Geometry: final body of the model. Coordinates: model frame, mm. Face numbers are marked on the shaded views. A direction names the side the tool comes from. Give positions to 0.01 mm unless a question says otherwise; leave off trailing zeros. Write each loop counter-clockwise with the first axis right and the second up, starting at its lowest first coordinate (ties: lowest second). Pieces come first, ordered by that corner, then holes.
Q1. Section C-C (y = 1.5). Return the cut outline in (x, z).
Q2. Mould query, pull axis X, two halves, no side actions, for the marked faces 6, 7, 8 and 9. Classes: +X half, -X half, draft (parallel to the pull), parting line (faces both ways), or undercut.
Q3. Section B-B (x = 3.5). Return the cut outline in (y, z), plus the area to 3 significant figures.
Q4. Section D-D (x = 18.5). Return the cut outline in (y, z), plus the area to 3 significant figures.
Q5. Line query: line 1 (Y direction, x = -9, z = 5.5); line 2 (X direction, y = -7, z = 0.25); line 3 (X direction, y = -10, z = 3.25). Output: solid intervals per line, ascending.
Q6. Pin query (flat end, axial travel): pin 1 Ø1 at (x, z) = (25.5, 3.5) entering from +Y; pin 2 Ø2 at (y, z) = (-25.5, -0.5) entering from -X; pin 3 Ø10 at (x, z) = (-21.5, 5) entering from -Y. Return the tip coordinate at first contact, or that it passes through.
Q7. Section A-A (z = 3.5). Return the cut outline in (x, y), plus the area to 3 significant figures.
Q8. Reachability of the marked faces 1, 2, 3, 4 and 5 from +Z, -Z, +X, -X, +Y, -Y: full face, straight path, thin tool, end or side. Return the list, or none.
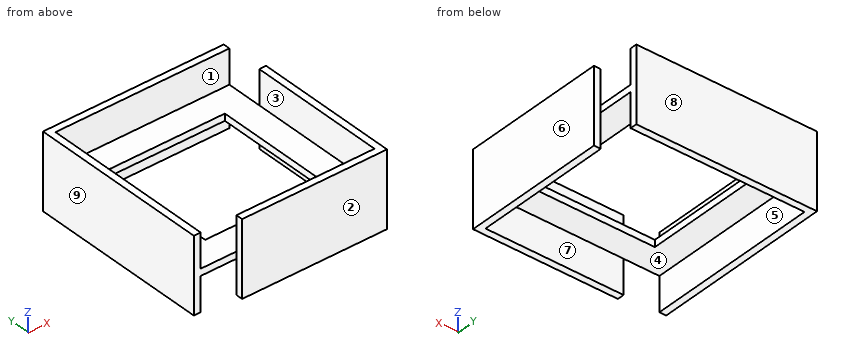
from build123d import *

# Parameters (mm, degrees)
F1_DEPTH = 12
F0_W     = 35
F0_H     = 35
F2_DEPTH = 2
F0_R     = 5
F3_DEPTH = 10


with BuildPart() as f1:
    # F0 (on Top) → F1 (new body)
    with BuildSketch(Plane.XY):
        Polygon((24.28125, 28.71875), (-28.71875, 28.71875), (-28.71875, -24.28125), (-26.71875, -24.28125), (-26.71875, 26.71875), (24.28125, 26.71875), align=None)
    extrude(amount=F1_DEPTH)



with BuildPart() as f1b:
    # F0 (on Top) → F1, piece 2 (new body)
    with BuildSketch(Plane.XY):
        Polygon((26.28125, -26.28125), (26.28125, 16.21875), (24.28125, 16.21875), (24.28125, -24.28125), (-16.21875, -24.28125), (-16.21875, -26.28125), align=None)
    extrude(amount=F1_DEPTH)


with BuildPart() as f1_1:
    add(f1.part)

    add(f1b.part)  # F2 merges F1b
    # F0 (on Top) → F2 (join)
    with BuildSketch(Plane.XY):
        Polygon((24.28125, 18.71875), (24.28125, 26.71875), (-26.71875, 26.71875), (-26.71875, -24.28125), (-18.71875, -24.28125), (-16.21875, -24.28125), (24.28125, -24.28125), (24.28125, 16.21875), align=None)
        with Locations((-1.21875, 1.21875)):
            Rectangle(F0_W, F0_H, mode=Mode.SUBTRACT)
    extrude(amount=F2_DEPTH)

    # F0 (on Top) → F3 (join)
    with BuildSketch(Plane.XY):
        Polygon((24.28125, 28.71875), (-28.71875, 28.71875), (-28.71875, -24.28125), (-26.71875, -24.28125), (-26.71875, 26.71875), (24.28125, 26.71875), align=None)
        Polygon((26.28125, -26.28125), (26.28125, 16.21875), (24.28125, 16.21875), (24.28125, -24.28125), (-16.21875, -24.28125), (-16.21875, -26.28125), align=None)
    extrude(amount=-F3_DEPTH)


with BuildPart() as f2:
    # F0 (on Top) → F2, piece 2 (new body)
    with BuildSketch(Plane.XY):
        with Locations((-1.21875, 1.21875)):
            Circle(F0_R)
    extrude(amount=F2_DEPTH)


solid = f1_1.part
Computed:
1. outline: (-28.72, -10) - (-26.72, -10) - (-26.72, 0) - (-18.72, 0) - (-18.72, 2) - (-26.72, 2) - (-26.72, 12) - (-28.72, 12) - close; (16.28, 0) - (24.28, 0) - (24.28, -10) - (26.28, -10) - (26.28, 12) - (24.28, 12) - (24.28, 2) - (16.28, 2) - close
2. face 6: +X half
2. face 7: undercut
2. face 8: draft
2. face 9: -X half
3. outline: (-26.28, -10) - (-24.28, -10) - (-24.28, 0) - (-16.28, 0) - (-16.28, 2) - (-24.28, 2) - (-24.28, 12) - (-26.28, 12) - close; (18.72, 0) - (26.72, 0) - (26.72, -10) - (28.72, -10) - (28.72, 12) - (26.72, 12) - (26.72, 2) - (18.72, 2) - close
3. area: 120 mm2
4. outline: (-26.28, -10) - (-24.28, -10) - (-24.28, 0) - (26.72, 0) - (26.72, -10) - (28.72, -10) - (28.72, 12) - (26.72, 12) - (26.72, 2) - (-24.28, 2) - (-24.28, 12) - (-26.28, 12) - close
4. area: 190 mm2
5. line 1: y = -26.28 to -24.28, 26.72 to 28.72
5. line 2: x = -28.72 to -18.72, 16.28 to 26.28
5. line 3: x = -28.72 to -26.72, 24.28 to 26.28
6. pin 1: stops at y = 16.22
6. pin 2: stops at x = -16.22
6. pin 3: stops at y = -24.28
7. outline: (-28.72, -24.28) - (-26.72, -24.28) - (-26.72, 26.72) - (24.28, 26.72) - (24.28, 28.72) - (-28.72, 28.72) - close; (-16.22, -26.28) - (26.28, -26.28) - (26.28, 16.22) - (24.28, 16.22) - (24.28, -24.28) - (-16.22, -24.28) - close
7. area: 374 mm2
8. face 1: +Z, +X
8. face 2: +Z, -Z, +X, -X, -Y
8. face 3: +Z
8. face 4: -Z
8. face 5: -Z, -Y
